Build history of the part. All positions in model axes, mm. Round coordinates to 2 decimals unless told otherwise and drop trailing zeros. Order: outer loops, then holes, each group sorted by start corner. A loop starts at its lowest first (then second) coordinate and runs counter-clockwise, first axis right, second up. Notation, with made-up numbers: (75, 83) -> (128, 83) arc R5 ccw to (128, 87) -> close; hole circle Ø10 at (21, 68). An arc over 180 degrees is marked (long way). Write item = value, one per line.
from build123d import *

# Parameters (mm, degrees)
F0_W     = 23.25
F0_H     = 69.75
F0_R     = 5
F1_DEPTH = 2.33
F2_R     = 11.62499


# Not quite as in the source:
# - a fillet or chamfer is up to 0.001 mm smaller than in the source, because OpenCascade refuses the exact size


with BuildPart() as f1:
    # F0 (on Top) → F1 (new body)
    with BuildSketch(Plane.XY):
        with Locations((11.625, 34.875)):
            Rectangle(F0_W, F0_H)
        with Locations((11.625, 58.125)):
            Circle(F0_R, mode=Mode.SUBTRACT)
    extrude(amount=F1_DEPTH)

    # F2 (radius 11.625 in the source; OpenCascade refuses exactly that, so slightly less here)
    f2_edges = [f1.edges().sort_by_distance(p)[0] for p in [
        (23.25, 0, 1.165),
        (0, 0, 1.165),
        (0, 69.75, 1.165),
        (23.25, 69.75, 1.165),
    ]]
    fillet(f2_edges, radius=F2_R)


solid = f1.part
Q1. Cut at C-C, the plane y = 9.5. List the corners of the cut face in (x, z), and give its area (3 significant figures).
Check values:
outline = (0.2, 0) -> (23.05, 0) -> (23.05, 2.33) -> (0.2, 2.33) -> close
area = 53.3 mm²
Q2. Probe probe 1 along Y at (x, z) = (12, 0.6); probe 2 along X at (y, z) = (57.5, 1.65); probe 3 along X at (y, z) = (56.5, 2.05). List the from-to ranges inside material, lowest first.
Check values:
probe_1 = 0.01 to 53.14, 63.11 to 69.74
probe_2 = 0 to 6.66, 16.59 to 23.25
probe_3 = 0 to 6.9, 16.35 to 23.25
Q3. Mould opens along Y. For faces 1 (the face through (19.75, 66.44, 1.18)), 2 (the face through (11, 35, 2.33)), 3 (the face through (14.313, 62.341, 1.149)) say: released by +Y, released by -Y, zero draft, split by the parting line, or undercut.
Check values:
face_1 = released by +Y
face_2 = zero draft
face_3 = undercut
Q4. Cut at B-B, the plane x = 3. List the corners of the cut face in (y, z).
Check values:
outline = (3.83, 0) -> (65.92, 0) -> (65.92, 2.33) -> (3.83, 2.33) -> close
